from build123d import *

# Parameters (mm, degrees)
SKIZZE1_W                       = 400
SKIZZE1_H                       = 170
AUFSATZ_LINEAR_AUSTRAGEN1_DEPTH = 5
SKIZZE3_W                       = 11.75
SKIZZE3_H                       = 11.75
SKIZZE3_R                       = 2.25
SKIZZE3_W_2                     = 11.5
SKIZZE3_H_2                     = 11.5
SKIZZE3_W_3                     = 23.5
SKIZZE3_W_4                     = 23.25
AUFSATZ_LINEAR_AUSTRAGEN6_DEPTH = 5
AUFSATZ_LINEAR_AUSTRAGEN7_DEPTH = 26
SKIZZE6_W                       = 160
SKIZZE6_H                       = 40
AUFSATZ_LINEAR_AUSTRAGEN8_DEPTH = 3


with BuildPart() as part:
    # Skizze1 → Aufsatz-Linear austragen1 (new body)
    with BuildSketch(Plane(origin=(0, 0, 0), x_dir=(1, 0, 0), z_dir=(0, 1, 0))):
        Rectangle(SKIZZE1_W, SKIZZE1_H)
    extrude(amount=AUFSATZ_LINEAR_AUSTRAGEN1_DEPTH)

    # Skizze3 → Aufsatz-Linear austragen6 (add)
    # profile 1 of 6: a face of its own
    with BuildSketch(Plane(origin=(0, 5, 0), x_dir=(1, 0, 0), z_dir=(0, 1, 0))):
        with Locations((74.125, 34.125)):
            Rectangle(SKIZZE3_W, SKIZZE3_H)
        with Locations(Location((75.75, 35.75, 0), (0, 0, 270))):
            Circle(SKIZZE3_R, mode=Mode.SUBTRACT)
    # profile 2 of 6: a face of its own
    with BuildSketch(Plane(origin=(0, 5, 0), x_dir=(1, 0, 0), z_dir=(0, 1, 0))):
        with Locations((-74.125, 34.125)):
            Rectangle(SKIZZE3_W, SKIZZE3_H)
        with Locations(Location((-75.75, 35.75, 0), (0, 0, 270))):
            Circle(SKIZZE3_R, mode=Mode.SUBTRACT)
    # profile 3 of 6: a face of its own
    with BuildSketch(Plane(origin=(0, 5, 0), x_dir=(1, 0, 0), z_dir=(0, 1, 0))):
        with Locations((-74.125, -34.125)):
            Rectangle(SKIZZE3_W, SKIZZE3_H)
        with Locations(Location((-75.75, -35.75, 0), (0, 0, 270))):
            Circle(SKIZZE3_R, mode=Mode.SUBTRACT)
    # profile 4 of 6: a face of its own
    with BuildSketch(Plane(origin=(0, 5, 0), x_dir=(1, 0, 0), z_dir=(0, 1, 0))):
        with Locations((74.25, -34.25)):
            Rectangle(SKIZZE3_W_2, SKIZZE3_H_2)
        with Locations(Location((76, -36, 0), (0, 0, 270))):
            Circle(SKIZZE3_R, mode=Mode.SUBTRACT)
    # profile 5 of 6: a face of its own
    with BuildSketch(Plane(origin=(0, 5, 0), x_dir=(1, 0, 0), z_dir=(0, 1, 0))):
        with Locations((0, -34.125)):
            Rectangle(SKIZZE3_W_3, SKIZZE3_H)
        with Locations(Location((-4.25, -35.75, 0), (0, 0, 270))):
            Circle(SKIZZE3_R, mode=Mode.SUBTRACT)
        with Locations(Location((4.25, -35.75, 0), (0, 0, 270))):
            Circle(SKIZZE3_R, mode=Mode.SUBTRACT)
    # profile 6 of 6: a face of its own
    with BuildSketch(Plane(origin=(0, 5, 0), x_dir=(1, 0, 0), z_dir=(0, 1, 0))):
        with Locations((0.125, 34.125)):
            Rectangle(SKIZZE3_W_4, SKIZZE3_H)
        with Locations(Location((-4.25, 35.75, 0), (0, 0, 270))):
            Circle(SKIZZE3_R, mode=Mode.SUBTRACT)
        with Locations(Location((4.25, 35.75, 0), (0, 0, 270))):
            Circle(SKIZZE3_R, mode=Mode.SUBTRACT)
    extrude(amount=AUFSATZ_LINEAR_AUSTRAGEN6_DEPTH)

    # Skizze4 → Aufsatz-Linear austragen7 (add)
    with BuildSketch(Plane(origin=(0, 5, 0), x_dir=(1, 0, 0), z_dir=(0, 1, 0))):
        Polygon((-83, 80), (-83, -40), (-80, -40), (-80, -28.25), (-80, 28.25), (-80, 40), (-80, 80), align=None)
        Polygon((83, -40), (80, -40), (68.5, -40), (11.75, -40), (-11.75, -40), (-68.25, -40), (-80, -40), (-83, -40), (-83, -43), (83, -43), align=None)
        Polygon((80, -28.5), (80, -40), (83, -40), (83, 80), (80, 80), (80, 40), (80, 28.25), align=None)
    extrude(amount=AUFSATZ_LINEAR_AUSTRAGEN7_DEPTH)

    # Skizze6 → Aufsatz-Linear austragen8 (add)
    with BuildSketch(Plane(origin=(0, 31, 0), x_dir=(1, 0, 0), z_dir=(0, 1, 0))):
        with Locations((0, 60)):
            Rectangle(SKIZZE6_W, SKIZZE6_H)
    extrude(amount=-AUFSATZ_LINEAR_AUSTRAGEN8_DEPTH)


solid = part.part
The model under review builds one solid part; all positions refer to its coordinate system, in mm. A direction names the side the tool comes from. Coordinates: 2 decimals unless noted, no trailing zeros. Write each loop counter-clockwise with the first axis right and the second up, starting at its lowest first coordinate (ties: lowest second). Pieces come first, ordered by that corner, then holes. Notation, with made-up numbers: (15, 4.25) - (70, 4.25) arc R21 cw to (70, 29.25) - close; hole circle Ø10 at (10, -6.5). An arc over 180 degrees is marked (long way). Answer as a JSON object with one key per item and string values. Group by question number.
1. Mouldability with a two-part tool opening along Z and no side actions: class faces 4 (the face through (-1, 18, 43)), 5 (the face through (19, 29, -80)), 6 (the face through (80, 18, -21)) as pulls with the +Z half, pulls with the -Z half, needs draft (parallel to the pull), parting line crosses it, or undercut.
2. Machinability: for faces 1 (the face through (83, 18, -18)), 2 (the face through (-83, 18, -19)), 3 (the face through (74, 10, 34)), which of the approach directions +Z, -Z, +X, -X, +Y, -Y give a long, thin tool a straight path to every point of the face, cutting with its end or side? Answer none if there is none.
3. Add section C-C (z = 18). Give the boundary of the cut face in (x, y), plus the area to 3 significant figures.
4. Add section A-A (y = 16). Give the boundary of the cut face in (x, z).
5. Clearance check with flat-ended pins moving along their axes: pin 1 Ø5 at (x, z) = (-75.5, -36.5) entering from +Y; pin 2 Ø6 at (x, z) = (-47.5, -55) entering from -Y; pin 3 Ø2.5 at (x, z) = (75.75, -35.75) entering from +Y; pin 4 Ø2.5 at (x, y) = (73.5, 8) entering from -Z. State where each tip first meets the part, or that it passes through.
6. Add section B-B (x = 22). Give the boundary of the cut face in (y, z).
7. To check wall thickness, follow probe 1 along X at (y, z) = (9, 29); probe 2 along X at (y, z) = (25, -23.5); probe 3 along Y at (x, z) = (-1, -75). State the ranges of each line that lie inside material, in increasing order.
8. Add section D-D (x = -104.5). Give the boundary of the cut face in (y, z), plus the area to 3 significant figures.
Findings:
{
 "1": {"face 4": "pulls with the +Z half", "face 5": "pulls with the -Z half", "face 6": "undercut"},
 "2": {"face 1": "+Z, -Z, +X, +Y", "face 2": "+Z, -Z, -X, +Y", "face 3": "-Z, +Y"},
 "3": {"outline": "(-200, 0) - (200, 0) - (200, 5) - (83, 5) - (83, 31) - (80, 31) - (80, 5) - (-80, 5) - (-80, 31) - (-83, 31) - (-83, 5) - (-200, 5) - close", "area": "2,160 mm²"},
 "4": {"outline": "(-83, -80) - (-80, -80) - (-80, 40) - (80, 40) - (80, -80) - (83, -80) - (83, 43) - (-83, 43) - close"},
 "5": {"pin 1": "y = 10", "pin 2": "y = 0", "pin 3": "y = 5", "pin 4": "z = -40"},
 "6": {"outline": "(0, -85) - (5, -85) - (5, 40) - (31, 40) - (31, 43) - (5, 43) - (5, 85) - (0, 85) - close; (28, -80) - (31, -80) - (31, -40) - (28, -40) - close"},
 "7": {"probe 1": "-83 to -68.25, -11.75 to 11.75, 68.5 to 83", "probe 2": "-83 to -80, 80 to 83", "probe 3": "0 to 5, 28 to 31"},
 "8": {"outline": "(0, -85) - (5, -85) - (5, 85) - (0, 85) - close", "area": "850 mm²"}
}
